from build123d import *

# Parameters (mm, degrees)
SKETCH043_R  = 3.8
PAD017_DEPTH = 1.4
SKETCH044_R  = 3.2
PAD018_DEPTH = 2.4
FILLET017_R  = 1


with BuildPart() as part:
    # Sketch043 → Pad017 (new body)
    with BuildSketch(Plane.XZ):
        with Locations((28.8, 9.2)):
            Circle(SKETCH043_R)
    extrude(amount=PAD017_DEPTH)

    # Sketch044 (on Face3 of Pad017) → Pad018 (join)
    with BuildSketch(Plane.XZ.offset(1.4)):
        with Locations((28.8, 9.2)):
            Circle(SKETCH044_R)
    extrude(amount=PAD018_DEPTH)

    # Fillet017
    fillet017_edges = [part.edges().sort_by_distance(p)[0] for p in [
        (25.6, -3.8, 9.2),
    ]]
    fillet(fillet017_edges, radius=FILLET017_R)


with BuildPart() as part_1:
    # Body005 placement: moved
    add(part.part.moved(Location((49, 0.6, 0))))


solid = part_1.part
Could you check a few things on this model? Use its own coordinates, in mm. A direction names the side the tool comes from. Coordinates: 2 decimals unless noted, no trailing zeros. Write each loop counter-clockwise with the first axis right and the second up, starting at its lowest first coordinate (ties: lowest second). Pieces come first, ordered by that corner, then holes. Notation, with made-up numbers: (-20.75, 0.5) - (-16.75, 0.5) arc R19 ccw to (-16.75, 4.5) - close; hole circle Ø7 at (42.25, 78). An arc over 180 degrees is marked (long way). Put each result on its own line as item: value. Start each with the question number.
Q1. I'm going to push a flat-ended pin straight in: P1, Ø4, axis at x = 75, z = 12, coming from the +Y side. Where does the tip first touch, or does it pass through?
Q2. I want a section at D-D on z = 12.5. Write out the boundary of the cut face in (x, y), plus the area to 3 significant figures.
Q3. I want a section at A-A on z = 9.2. Write out the boundary of the cut face in (x, y).
Q4. I want a section at B-B on x = 77.8. Write out the boundary of the cut face in (y, z), plus the area to 3 significant figures.
Q5. Please list where these lines run through material, in increasing order: L1, parallel to X at y = 0.05, z = 11.25; L2, parallel to Y at x = 76, z = 6.25; L3, parallel to Y at x = 80.75, z = 10.
Q6. I want a section at C-C on y = -2.1. Write out the boundary of the cut face in (x, z), plus the area to 3 significant figures.
Q7. Which directions (+Z, -Z, +X, -X, +Y, -Y) give clear straight access to the entire face, cutting with the end or side of a thin tool? Please do faces 1 (the cylindrical face through (75.44, -1.49, 11.36)), 2 (the flat face through (78, 0.6, 9)).
Checks:
1. P1: y = 0.6
2. outline: (75.92, -0.8) - (79.68, -0.8) - (79.68, 0.6) - (75.92, 0.6) - close
2. area: 5.28 mm²
3. outline: (74, -0.8) - (74.6, -0.8) - (74.6, -2.2) arc R1 ccw to (75.6, -3.2) - (80, -3.2) arc R1 ccw to (81, -2.2) - (81, -0.8) - (81.6, -0.8) - (81.6, 0.6) - (74, 0.6) - close
4. outline: (-3.2, 7) arc R1 ccw to (-2.2, 6) - (-0.8, 6) - (-0.8, 5.4) - (0.6, 5.4) - (0.6, 13) - (-0.8, 13) - (-0.8, 12.4) - (-2.2, 12.4) arc R1 ccw to (-3.2, 11.4) - close
4. area: 25.6 mm²
5. L1: 74.6 to 81
5. L2: -0.8 to 0.6
5. L3: -2.72 to 0.6
6. outline: circle Ø6.4 at (77.8, 9.2)
6. area: 32.2 mm²
7. face 1: -Y
7. face 2: +Z, -Z, +X, -X, +Y
